from build123d import *

# Parameters (mm, degrees)
F1_DEPTH = 8.1
F2_R     = 1.75
F3_DEPTH = 9.001
F4_R     = 1


with BuildPart() as f1:
    # F0 (on Front) → F1 (new body)
    with BuildSketch(Plane.XZ):
        Polygon((-8.6, 9), (-8.6, 0), (-3.55, 0), (-3.55, 4.5), (3.55, 4.5), (3.55, 0), (8.6, 0), (8.6, 9), align=None)
    extrude(amount=F1_DEPTH)

    # F2 (on face) → F3 (cut, through all)
    with BuildSketch(Plane.XY.offset(9)):
        with Locations((-5.575, -4.05)):
            Circle(F2_R)
        with Locations((5.575, -4.05)):
            Circle(F2_R)
    extrude(amount=-F3_DEPTH, mode=Mode.SUBTRACT)

    # F4
    f4_edges = [f1.edges().sort_by_distance(p)[0] for p in [
        (0, -8.1, 9),
        (0, 0, 9),
        (-3.55, -4.05, 4.5),
        (3.55, -4.05, 4.5),
    ]]
    fillet(f4_edges, radius=F4_R)


solid = f1.part
Work out the finished part from the listing and answer in its coordinate system (mm). A direction names the side the tool comes from. Coordinates: 2 decimals unless noted, no trailing zeros. Loops run counter-clockwise (first coordinate to the right, second up) from the corner with the lowest first, then second, coordinate; pieces in that order, holes last. Notation, with made-up numbers: M 63.5,72.25 L 97.5,72.25 A28 ccw 97.5,109.25 Z; hole C 41,82 d2. An arc over 180 degrees is marked long. Answer in a Markdown table with one row per item. Add a question column.
1. Find section D-D, the plane z = 4.75. Write down the section's boundary in (x, y) (3 decimals).
2. Flat-ended cylindrical pins translate along their axes: P1, Ø2, axis at x = -5.575, y = -4.05, coming from the -Z side; P2, Ø3, axis at x = -4, y = -3, coming from the -Z side. Find the tip coordinate at first contact, or state that the pin passes through.
3. Find section C-C, the plane x = 5. Write down the section's boundary in (y, z).
4. Find section B-B, the plane y = -4.05. Write down the section's boundary in (x, z) (3 decimals).
5. A tool of negligible diameter and unlimited length cuts with its end or side. For faces 4 (the flat face through (8, -4, 0)), 5 (the flat face through (-3.55, -4, 2)), from which of +Z, -Z, +X, -X, +Y, -Y can it reach the whole face along a straight path? Write none if from no direction.
6. The mould has two halves that part along X. Classify faces 1 (the cylindrical face through (-3.265, -4.107, 4.199)), 2 (the flat face through (-7.23, -3.09, 0)), 3 (the flat face through (-8.6, -4, 5)): pulls with the +X half, pulls with the -X half, needs draft (parallel to the pull), parting line crosses it, or undercut.
7. Find section A-A, the plane z = 2. Write down the section's boundary in (x, y) (3 decimals), then the cut area to 3 significant figures.
8. Consider L1, parallel to X at y = -4, z = 3; L2, parallel to X at y = -2.5, z = 8. Determine where each line is inside the solid, lowest interval first.
Reported:
| question | item | result |
|---|---|---|
| 1 | outline | M -8.6,-8.1 L 8.6,-8.1 L 8.6,0 L -8.6,0 Z; hole C -5.575,-4.05 d3.5; hole C 5.575,-4.05 d3.5 |
| 2 | P1 | passes through |
| 2 | P2 | stops at z = 0 |
| 3 | outline | M -8.1,0 L -5.7,0 L -5.7,9 L -7.1,9 A1 ccw -8.1,8 Z; M -2.4,0 L 0,0 L 0,8 A1 ccw -1,9 L -2.4,9 Z |
| 4 | outline | M -8.6,0 L -7.325,0 L -7.325,9 L -8.6,9 Z; M -3.825,0 L -3.55,0 L -3.55,3.5 A1 cw -2.55,4.5 L 2.55,4.5 A1 cw 3.55,3.5 L 3.55,0 L 3.825,0 L 3.825,9 L -3.825,9 Z; M 7.325,0 L 8.6,0 L 8.6,9 L 7.325,9 Z |
| 5 | face 4 | -Z, +X, -X, +Y, -Y |
| 5 | face 5 | -Z, +Y, -Y |
| 6 | face 1 | undercut |
| 6 | face 2 | needs draft |
| 6 | face 3 | pulls with the -X half |
| 7 | outline | M -8.6,-8.1 L -3.55,-8.1 L -3.55,0 L -8.6,0 Z; M 3.55,-8.1 L 8.6,-8.1 L 8.6,0 L 3.55,0 Z; hole C -5.575,-4.05 d3.5; hole C 5.575,-4.05 d3.5 |
| 7 | area | 62.6 mm^2 |
| 8 | L1 | x = -8.6 to -7.32, -3.83 to -3.55, 3.55 to 3.83, 7.32 to 8.6 |
| 8 | L2 | x = -8.6 to -6.39, -4.76 to 4.76, 6.39 to 8.6 |
